Drawing for the job (mm, zero at the part's lowest x, y, z). A direction names the side the tool comes from. Give positions to 0.01 mm unless a question says otherwise; leave off trailing zeros. Loops run counter-clockwise (first coordinate to the right, second up) from the corner with the lowest first, then second, coordinate; pieces in that order, holes last.
1) Band-saw the part on C-C on y = 8. List the corners of the cut face in (x, z).
2) Two-plate mould, pull along X, no slides. Class the marked faces 1, 2 and 3: +X half, -X half, draft (parallel to the pull), parting line (faces both ways), or undercut.
3) Band-saw the part on D-D on z = 15. List the corners of the cut face in (x, y), then the cut area to 3 significant figures.
4) Wall check: line 1 (Z direction, x = 17, y = 4.7); line 2 (X direction, y = 4.6, z = 15); line 3 (X direction, y = 6.5, z = 28.8). Give the ranges that are in metal, low to high.
5) Band-saw the part on B-B on x = 17. List the corners of the cut face in (y, z).
6) Band-saw the part on A-A on z = 28.8. List the corners of the cut face in (x, y).
7) Flat gauge pins, fed straight in: P1, Ø2.5, axis at x = 15, z = 15.5, coming from the +Y side; P2, Ø2, axis at x = 16.5, y = 5.5, coming from the -Z side; P3, Ø2, axis at x = 3.5, y = 4.5, coming from the +Z side. Where does each tip first touch, or does it go through?
8) 3-axis set-ups, long thin cutter, end or side, ignore diameter. For the marked faces 4, 5 and 6: which of +Z, -Z, +X, -X, +Y, -Y reach the whole face in a straight line?
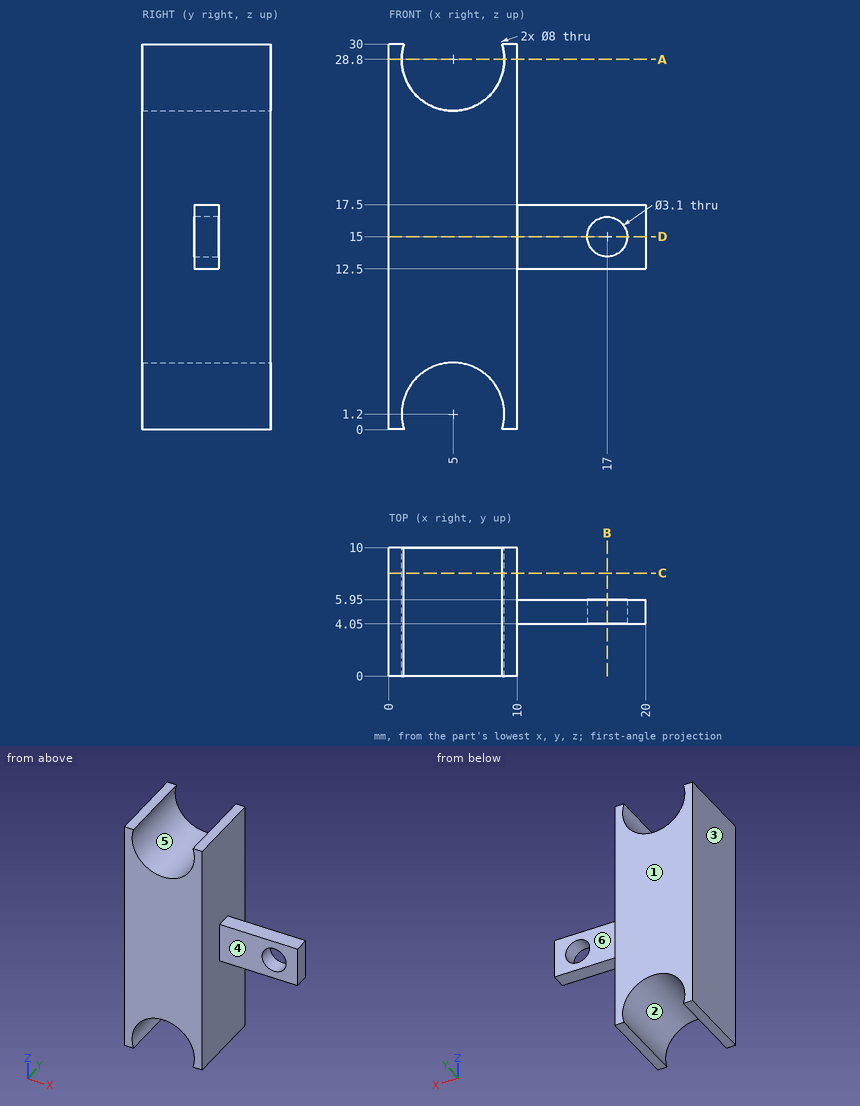
Findings below:
1. outline: (0, 0) - (1.18, 0) arc R4 cw (long way) to (8.82, 0) - (10, 0) - (10, 30) - (8.82, 30) arc R4 cw (long way) to (1.18, 30) - (0, 30) - close
2. face 1: draft
2. face 2: undercut
2. face 3: -X half
3. outline: (0, 0) - (10, 0) - (10, 4.05) - (15.45, 4.05) - (15.45, 5.95) - (10, 5.95) - (10, 10) - (0, 10) - close; (18.55, 4.05) - (20, 4.05) - (20, 5.95) - (18.55, 5.95) - close
3. area: 113 mm2
4. line 1: z = 12.5 to 13.45, 16.55 to 17.5
4. line 2: x = 0 to 15.45, 18.55 to 20
4. line 3: x = 0 to 1, 9 to 10
5. outline: (4.05, 12.5) - (5.95, 12.5) - (5.95, 13.45) - (4.05, 13.45) - close; (4.05, 16.55) - (5.95, 16.55) - (5.95, 17.5) - (4.05, 17.5) - close
6. outline: (0, 0) - (1, 0) - (1, 10) - (0, 10) - close; (9, 0) - (10, 0) - (10, 10) - (9, 10) - close
7. P1: stops at y = 5.95
7. P2: stops at z = 12.5
7. P3: stops at z = 25.68
8. face 4: +Z, -Z, +X, -Y
8. face 5: +Y, -Y
8. face 6: +Z, -Z, +X, +Y
